The listing builds one solid part. Answer for the finished solid, in the listing's coordinates (mm). A direction names the side the tool comes from. Round coordinates to 2 decimals unless told otherwise and drop trailing zeros. Loops run counter-clockwise (first coordinate to the right, second up) from the corner with the lowest first, then second, coordinate; pieces in that order, holes last. Notation, with made-up numbers: M -22,-4.5 L -2,-4.5 A12 ccw -2,5.5 Z; hole C 75,-6 d3. An arc over 180 degrees is marked long. Answer as a JSON object with one key per item and string values.
```python
from build123d import *

# Parameters (mm, degrees)
RESSALTO_EXTRUS_O1_DEPTH   = 6
RESSALTO_EXTRUS_O1_2_DEPTH = 6
RESSALTO_EXTRUS_O2_START   = 1
RESSALTO_EXTRUS_O2_DEPTH   = 2
RESSALTO_EXTRUS_O4_START   = 1
ESBO_O3_W                  = 30
ESBO_O3_H                  = 3
RESSALTO_EXTRUS_O4_DEPTH   = 1
ESBO_O5_W                  = 4
ESBO_O5_H                  = 26
RESSALTO_EXTRUS_O6_DEPTH   = 2
RESSALTO_EXTRUS_O7_DEPTH   = 15
FILETE7_R                  = 2
FILETE8_R                  = 0.5
FILETE9_R                  = 2


with BuildPart() as part:
    # Esbo_o1 → Ressalto-extrus_o1 (new, symmetric)
    with BuildSketch(Plane.XY):
        with BuildLine():
            Line((-9, -1.5), (9, -1.5))
            ThreePointArc((9, -1.5), (12, -4.5), (15, -1.5))
            Line((15, -1.5), (15, 1.5))
            Line((15, 1.5), (15, 7.918286702))
            ThreePointArc((15, 7.918286702), (1.876188275, 3.126620802), (-12, 1.5))
            ThreePointArc((-12, 1.5), (-14.121320344, 0.621320344), (-15, -1.5))
            ThreePointArc((-15, -1.5), (-12, -4.5), (-9, -1.5))
        make_face()
    extrude(amount=RESSALTO_EXTRUS_O1_DEPTH, both=True)



with BuildPart() as body_2:
    # Esbo_o1 → Ressalto-extrus_o1 2 (new, symmetric)
    with BuildSketch(Plane.XY):
        with BuildLine():
            Line((15, -25.142315596), (-15, -25.142315596))
            Line((-15, -25.142315596), (-15, -22.142315596))
            Line((-15, -22.142315596), (-3.5, -22.142315596))
            Line((-3.5, -22.142315596), (3.174548445, -22.142315596))
            Line((3.174548445, -22.142315596), (3.174548445, -16.732050808))
            Line((3.174548445, -16.732050808), (4.242268465, -16.732050808))
            ThreePointArc((4.242268465, -16.732050808), (5.462746803, -19.00323777), (7.90754076, -18.184189481))
            ThreePointArc((7.90754076, -18.184189481), (5.745986772, -13.568824016), (1.75, -16.732050808))
            ThreePointArc((1.75, -16.732050808), (-1, -19.482050808), (-3.75, -16.732050808))
            Line((-3.75, -16.732050808), (-3.75, -11))
            Line((-3.75, -11), (-0.75, -10))
            Line((-0.75, -10), (-0.75, -11))
            Line((-0.75, -11), (-0.75, -15))
            ThreePointArc((-0.75, -15), (-2.322875656, -17.877694731), (0.75, -16.732050808))
            ThreePointArc((0.75, -16.732050808), (6.283199983, -12.680397095), (8.475128378, -19.17867762))
            ThreePointArc((8.475128378, -19.17867762), (6.683061453, -20.158063602), (4.674548445, -19.788501348))
            Line((4.674548445, -19.788501348), (4.674548445, -22.142315596))
            Line((4.674548445, -22.142315596), (15, -22.142315596))
            Line((15, -22.142315596), (15, -25.142315596))
        make_face()
    extrude(amount=RESSALTO_EXTRUS_O1_2_DEPTH, both=True)


with BuildPart() as body_3:
    # Esbo_o2 → Ressalto-extrus_o2 (new body)
    with BuildSketch(Plane.XY.offset(6).offset(RESSALTO_EXTRUS_O2_START)):
        with BuildLine():
            Line((-15, -25.142315596), (15, -25.142315596))
            Line((15, -25.142315596), (15, 0.857684404))
            Line((15, 0.857684404), (-13, 0.857684404))
            ThreePointArc((-13, 0.857684404), (-14.414213562, 0.271897966), (-15, -1.142315596))
            Line((-15, -1.142315596), (-15, -25.142315596))
        make_face()
        with BuildLine():
            Line((-1, -12), (-1, -18))
            ThreePointArc((-1, -18), (-2.5, -19.5), (-4, -18))
            Line((-4, -18), (-4, -12))
            ThreePointArc((-4, -12), (-2.5, -10.5), (-1, -12))
        make_face(mode=Mode.SUBTRACT)
    extrude(amount=RESSALTO_EXTRUS_O2_DEPTH)


with BuildPart() as part_1:
    add(part.part)

    add(body_2.part)  # Ressalto-extrus_o4 merges body 2

    add(body_3.part)  # Ressalto-extrus_o4 merges body 3
    # Esbo_o3 → Ressalto-extrus_o4 (add)
    with BuildSketch(Plane.XY.offset(6).offset(RESSALTO_EXTRUS_O4_START)):
        with Locations((0, -23.642315596)):
            Rectangle(ESBO_O3_W, ESBO_O3_H)
        with BuildLine():
            Line((15, -1.5), (15, 7.918286702))
            ThreePointArc((15, 7.918286702), (1.876188275, 3.126620802), (-12, 1.5))
            ThreePointArc((-12, 1.5), (-14.121320344, -3.621320344), (-9, -1.5))
            Line((-9, -1.5), (9, -1.5))
            ThreePointArc((9, -1.5), (12, -4.5), (15, -1.5))
        make_face()
    extrude(amount=-RESSALTO_EXTRUS_O4_DEPTH)

    # Esbo_o5 → Ressalto-extrus_o6 (add)
    with BuildSketch(Plane(origin=(0, 0, -6), x_dir=(-1, 0, 0), z_dir=(0, 0, -1))):
        with Locations((-13, -12.142315596)):
            Rectangle(ESBO_O5_W, ESBO_O5_H)
        with BuildLine():
            Line((6.25, -25.142315596), (6.25, 0.857684404))
            Line((6.25, 0.857684404), (12.25, 0.857684404))
            ThreePointArc((12.25, 0.857684404), (14.194543648, 0.052228052), (15, -1.892315596))
            Line((15, -1.892315596), (15, -25.142315596))
            Line((15, -25.142315596), (6.25, -25.142315596))
        make_face()
    extrude(amount=-RESSALTO_EXTRUS_O6_DEPTH)

    # Esbo_o4 → Ressalto-extrus_o7 (add)
    with BuildSketch(Plane.XY.offset(6)):
        with BuildLine():
            Line((-1.3, -12), (-1.3, -13.5))
            ThreePointArc((-1.3, -13.5), (-2.5, -14.7), (-3.7, -13.5))
            Line((-3.7, -13.5), (-3.7, -12))
            ThreePointArc((-3.7, -12), (-2.5, -10.8), (-1.3, -12))
        make_face()
    extrude(amount=RESSALTO_EXTRUS_O7_DEPTH)

    # Filete7
    filete7_edges = [part_1.edges().sort_by_distance(p)[0] for p in [
        (4.674548445, -22.142315596, 0),
        (3.174548445, -22.142315596, 0),
    ]]
    fillet(filete7_edges, radius=FILETE7_R)

    # Filete8
    filete8_edges = [part_1.edges().sort_by_distance(p)[0] for p in [
        (4.242268465, -16.732050808, 0),
        (3.174548445, -16.732050808, 0),
    ]]
    fillet(filete8_edges, radius=FILETE8_R)

    # Filete9
    filete9_edges = [part_1.edges().sort_by_distance(p)[0] for p in [
        (-0.75, -15, 0),
    ]]
    fillet(filete9_edges, radius=FILETE9_R)


solid = part_1.part
```
Item 1: Flat-ended cylindrical pins translate along their axes: P1, Ø16.5, axis at x = 2, y = -8, coming from the -Z side; P2, Ø1.5, axis at y = -18.5, z = 3.5, coming from the -X side; P3, Ø2, axis at y = -12, z = 13, coming from the +X side; P4, Ø4, axis at y = -17, z = -1.5, coming from the +X side. Find the tip coordinate at first contact, or state that the pin passes through.
Values follow:
{"P1": "z = -6", "P2": "x = -3.55", "P3": "x = -1.3", "P4": "x = 9.25"}
Item 2: Determine the mould class of faces 5 (the face through (1, 0.858, 8)), 6 (the face through (5.66, -19.07, 0.08)), 7 (the face through (-15, -15, -5)) for opening direction Y: released by +Y, released by -Y, zero draft, split by the parting line, or undercut.
Values follow:
{"face 5": "released by +Y", "face 6": "undercut", "face 7": "zero draft"}
Item 3: The part is cut by section D-D (z = 11.75). Give the vertices of the cut face in (x, y).
Values follow:
{"outline": "M -3.7,-13.5 A1.2 ccw -1.3,-13.5 L -1.3,-12 A1.2 ccw -3.7,-12 Z"}
Item 4: The part is cut by section B-B (z = 6.5). Give the vertices of the cut face in (x, y), then the cut area to 3 significant figures.
Values follow:
{"outline": "M -15,-25.14 L 15,-25.14 L 15,-22.14 L -15,-22.14 Z; M -12,1.5 A3 ccw long -9,-1.5 L 9,-1.5 A3 ccw 15,-1.5 L 15,7.92 A60 cw Z; M -3.7,-13.5 A1.2 ccw -1.3,-13.5 L -1.3,-12 A1.2 ccw -3.7,-12 Z", "area": "271 mm^2"}
Item 5: Which of the six approach directions +Z, -Z, +X, -X, +Y, -Y give full straight-line access (tool end or side, diameter ignored) to faces 1 (the face through (-14.399, 0.287, 7.986)), 2 (the face through (11, -13, -5)), 3 (the face through (-2.5, -10.8, 13.4)), 4 (the face through (-4, -15, 8))?
Values follow:
{"face 1": "+Z, -X, +Y", "face 2": "-Z", "face 3": "+Z", "face 4": "+Z, -Z"}
Item 6: Straight lines are drawn through the part: line 1 (Z direction, x = 4.5, y = -22); line 2 (Z direction, x = -7, y = -17); line 3 (Y direction, x = -1, z = -2). For each, find the intervals that lie inside material, in ascending order.
Values follow:
{"line 1": "-6 to 6, 7 to 9", "line 2": "-6 to -4, 7 to 9", "line 3": "-25.14 to -22.14, -19.48 to -18.48, -14.38 to -10.08, -1.5 to 2.52"}
Item 7: The part is cut by section C-C (x = 11.5). Give the vertices of the cut face in (y, z).
Values follow:
{"outline": "M -25.14,-6 L 6.29,-6 L 6.29,7 L 0.86,7 L 0.86,9 L -25.14,9 Z; hole M -22.14,-4 L -4.46,-4 L -4.46,7 L -22.14,7 Z"}
